```python
from build123d import *

# Parameters (mm, degrees)
SKETCH_1_R      = 1.65
EXTRUDE_1_DEPTH = 2


with BuildPart() as part:
    # 草图1 → 凸台-拉伸1 (new body)
    with BuildSketch(Plane.XY):
        with BuildLine():
            Line((-37.605189444, 14.746778458), (-47.605189444, -2.573729618))
            Line((-47.605189444, -2.573729618), (38.997350935, -52.573729618))
            Line((38.997350935, -52.573729618), (48.997350935, -35.253221542))
            Line((48.997350935, -35.253221542), (14.191892619, -15.158280815))
            Line((14.191892619, -15.158280815), (-27.605658614, 57.237201553))
            Line((-27.605658614, 57.237201553), (-44.926166689, 47.237201553))
            Line((-44.926166689, 47.237201553), (-29.779250551, 21.001973223))
            ThreePointArc((-29.779250551, 21.001973223), (-30.573843664, 14.966439317), (-36.60937757, 14.171846204))
            Line((-36.60937757, 14.171846204), (-37.605189444, 14.746778458))
        make_face()
        with Locations((21.870944537, -31.13878889)):
            Circle(SKETCH_1_R, mode=Mode.SUBTRACT)
        with Locations((4.550436462, -21.13878889)):
            Circle(SKETCH_1_R, mode=Mode.SUBTRACT)
        with Locations((-12.770071614, -11.13878889)):
            Circle(SKETCH_1_R, mode=Mode.SUBTRACT)
        with Locations((-18.117652306, 20.803492565)):
            Circle(SKETCH_1_R, mode=Mode.SUBTRACT)
        with Locations((-23.117652306, 29.463746603)):
            Circle(SKETCH_1_R, mode=Mode.SUBTRACT)
        with Locations((-28.117652306, 38.124000641)):
            Circle(SKETCH_1_R, mode=Mode.SUBTRACT)
    extrude(amount=EXTRUDE_1_DEPTH)


solid = part.part
```
Verification items for the finished model (mm, model axes). A direction names the side the tool comes from. Give positions to 0.01 mm unless a question says otherwise; leave off trailing zeros. Order: outer loops, then holes, each group sorted by start corner. A loop starts at its lowest first (then second) coordinate and runs counter-clockwise, first axis right, second up. Notation, with made-up numbers: M 40,61.25 L 90,61.25 A27 cw 90,82.25 Z; hole C 33,-10 d10. An arc over 180 degrees is marked long. Return JSON: item names as keys, results as strings. Group by question number.
1) Section check D-D on x = 1. Record the cut outline in (y, z).
2) Section check A-A on x = -33. Record the cut outline in (y, z).
3) Mould release check, pull along X, two halves, no side actions. Record for faces 3 (the face through (-7, -1, 0)), 4 (the face through (43.93, -44.03, 0.99)), 5 (the face through (-30.51, 15.03, 0.99)), 6 (the face through (-4.91, -27.224, 0.986)): pulls with the +X half, pulls with the -X half, needs draft (parallel to the pull), parting line crosses it, or undercut.
4) Access from +Z, -Z, +X, -X, +Y, -Y to the whole of each face (thin tool, end or side, straight path). Record for faces 1 (the face through (31.838, -25.346, 0.986)), 2 (the face through (-42.535, 6.208, 0.986)).
5) Go/stop test with flat-tipped pins: pin 1 Ø2 at (x, y) = (-23.12, 29.46) entering from +Z; pin 2 Ø1 at (y, z) = (-40, 0.5) entering from -X; pin 3 Ø5.5 at (x, y) = (-18.12, 20.8) entering from +Z. Record where each tip stops, or that it passes through.
6) Scan lines: line 1 (Y direction, x = -13, z = 0.8); line 2 (Y direction, x = -30, z = 1.1); line 3 (X direction, y = -4.5, z = 1.65). Record each from-to range of solid material in increasing order.
7) Section check C-C on y = 41. Record the cut outline in (x, z).
8) Section check B-B on z = 0.5. Record the cut outline in (x, y), and give its area (3 significant figures).
Answer block:
{
 "1": {"outline": "M -30.64,0 L 7.69,0 L 7.69,2 L -30.64,2 Z"},
 "2": {"outline": "M -11.01,0 L 13.63,0 L 13.63,2 L -11.01,2 Z; M 26.58,0 L 54.12,0 L 54.12,2 L 26.58,2 Z"},
 "3": {"face 3": "needs draft", "face 4": "pulls with the +X half", "face 5": "undercut", "face 6": "pulls with the -X half"},
 "4": {"face 1": "+Z, -Z, +X, +Y", "face 2": "+Z, -Z, -X"},
 "5": {"pin 1": "passes through", "pin 2": "stops at x = 16.35", "pin 3": "stops at z = 2"},
 "6": {"line 1": "y = -22.55 to -12.77, -9.5 to 31.94", "line 2": "y = -12.74 to 15.65, 21.38 to 55.85", "line 3": "x = -44.27 to 8.04"},
 "7": {"outline": "M -41.33,0 L -18.23,0 L -18.23,2 L -41.33,2 Z"},
 "8": {"outline": "M -47.61,-2.57 L 39,-52.57 L 49,-35.25 L 14.19,-15.16 L -27.61,57.24 L -44.93,47.24 L -29.78,21 A5 cw -36.61,14.17 L -37.61,14.75 Z; hole C -28.12,38.12 d3.3; hole C -23.12,29.46 d3.3; hole C -18.12,20.8 d3.3; hole C -12.77,-11.14 d3.3; hole C 4.55,-21.14 d3.3; hole C 21.87,-31.14 d3.3", "area": "3,330 mm^2"}
}
